Geometry: see drawing. Coordinates: mm, zero at the bounding-box minimum. Coordinates: 2 decimals unless noted, no trailing zeros. Write each loop counter-clockwise with the first axis right and the second up, starting at its lowest first coordinate (ties: lowest second). Pieces come first, ordered by that corner, then holes.
1) Section query C-C (x = 3.5). Output: boundary loops of the cut face in (y, z).
2) Line query: L1, parallel to X at y = 3.25, z = 0.15; L2, parallel to Y at x = 4.5, z = 0.15; L3, parallel to X at y = 6.75, z = 0.05 (1 decimal). Output: solid intervals per line, ascending.
3) Section query A-A (y = 6). Output: boundary loops of the cut face in (x, z).
4) Section query B-B (z = 0.15). State how many separate pieces and enclosed holes the cut face has.
5) Section query D-D (y = 2). Output: boundary loops of the cut face in (x, z).
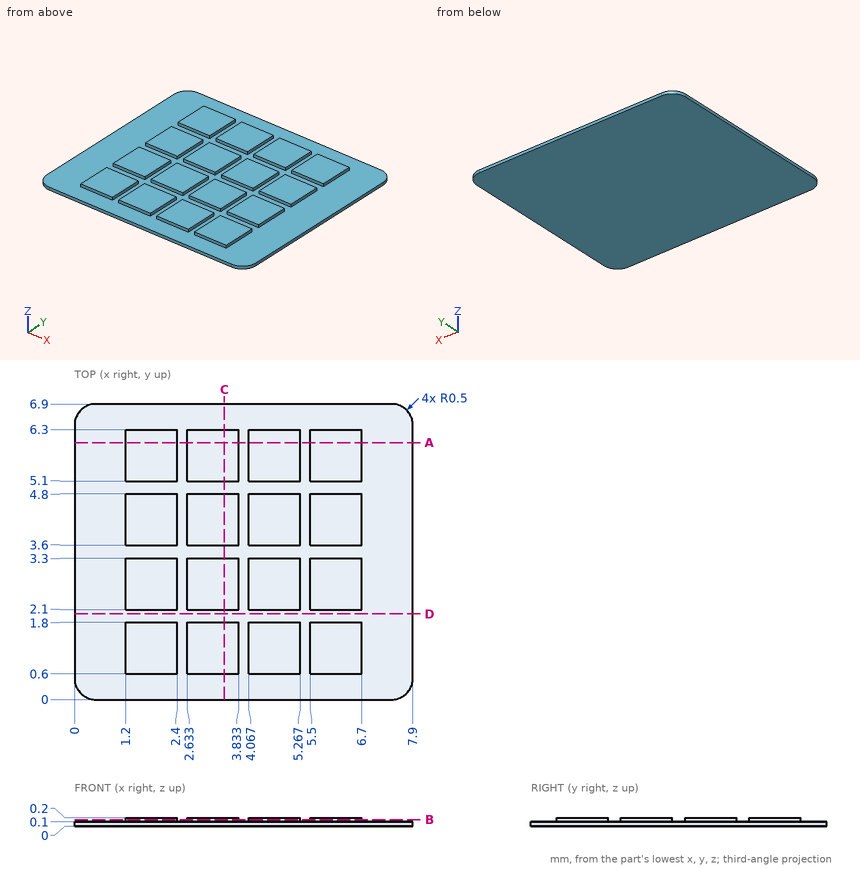
Answer:
1. outline: (0, 0) - (6.9, 0) - (6.9, 0.1) - (6.3, 0.1) - (6.3, 0.2) - (5.1, 0.2) - (5.1, 0.1) - (4.8, 0.1) - (4.8, 0.2) - (3.6, 0.2) - (3.6, 0.1) - (3.3, 0.1) - (3.3, 0.2) - (2.1, 0.2) - (2.1, 0.1) - (1.8, 0.1) - (1.8, 0.2) - (0.6, 0.2) - (0.6, 0.1) - (0, 0.1) - close
2. L1: x = 1.2 to 2.4, 2.63 to 3.83, 4.07 to 5.27, 5.5 to 6.7
2. L2: y = 0.6 to 1.8, 2.1 to 3.3, 3.6 to 4.8, 5.1 to 6.3
2. L3: x = 0.1 to 7.8
3. outline: (0, 0) - (7.9, 0) - (7.9, 0.1) - (6.7, 0.1) - (6.7, 0.2) - (5.5, 0.2) - (5.5, 0.1) - (5.27, 0.1) - (5.27, 0.2) - (4.07, 0.2) - (4.07, 0.1) - (3.83, 0.1) - (3.83, 0.2) - (2.63, 0.2) - (2.63, 0.1) - (2.4, 0.1) - (2.4, 0.2) - (1.2, 0.2) - (1.2, 0.1) - (0, 0.1) - close
4. separate pieces: 16
4. enclosed holes: 0
5. outline: (0, 0) - (7.9, 0) - (7.9, 0.1) - (0, 0.1) - close
